Part print with two shaded views. Sizes in mm from the minimum x, y, z corner. Give positions to 0.01 mm unless a question says otherwise; leave off trailing zeros. Loops run counter-clockwise (first coordinate to the right, second up) from the corner with the lowest first, then second, coordinate; pieces in that order, holes last. Notation, with made-up numbers: M -38.75,-20 L -26.75,-20 A19 ccw -26.75,-12 Z; hole C 29.5,50 d6. An arc over 180 degrees is marked long. Answer as a JSON object with one key per item and string values. Group by question number.
1. Mould opens along X. For the marked faces 1, 2 and 3 say: released by +X, released by -X, zero draft, split by the parting line, or undercut.
2. Drop a flat-ended pin along its axis: pin 1 Ø1.5 at (x, y) = (3.5, 55) entering from -Z. Give the stop position or say it passes through.
3. Slice it at D-D (x = 3). List the corners of the cut face in (y, z).
4. Slice it at C-C (x = 6). List the corners of the cut face in (y, z).
5. Slice it at A-A (y = 66). List the corners of the cut face in (x, z).
6. Slice it at B-B (z = 5.2). List the corners of the cut face in (x, y), then the cut area to 3 significant figures.
7. Drill centre lines: line 1 along Y through (x, z) = (6, 2); line 2 along Y through (x, z) = (4, 1.25); line 3 along X through (y, z) = (66, 4.25). Where is each one in solid material? Low to high. Write a range as [from, to].
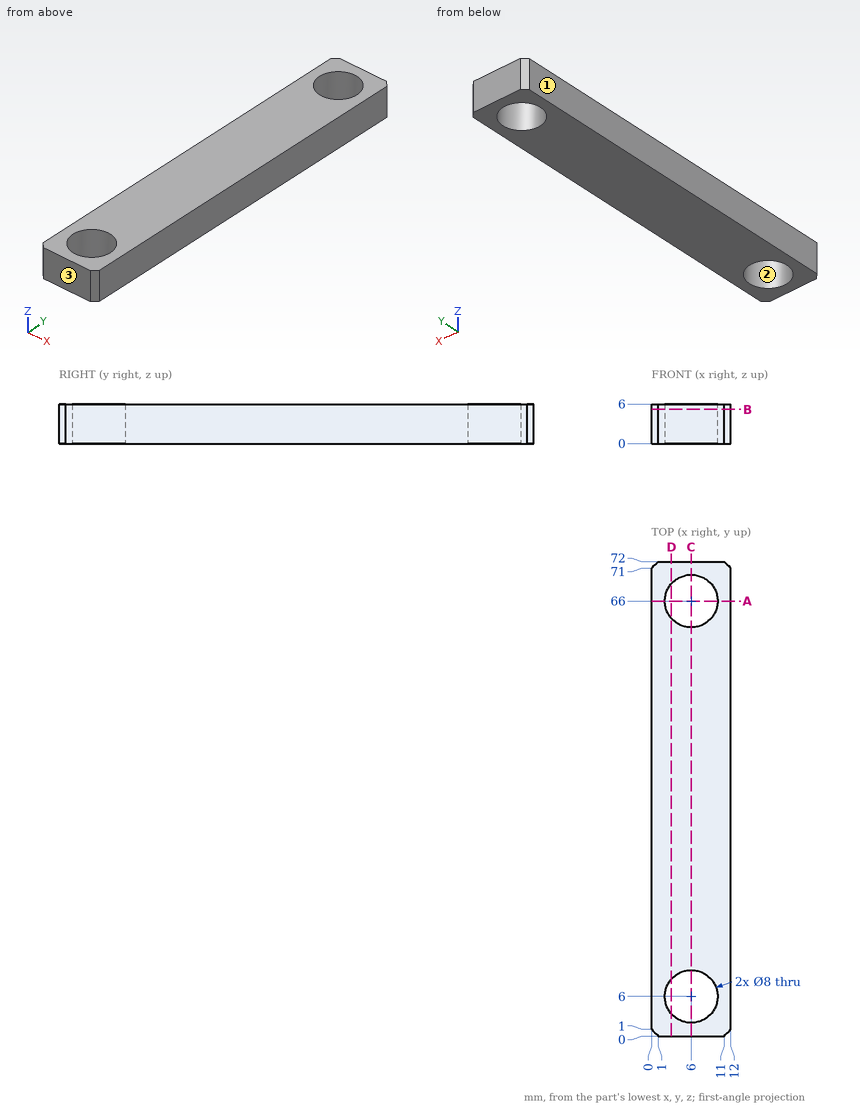
Established:
{
 "1": {"face 1": "released by -X", "face 2": "undercut", "face 3": "zero draft"},
 "2": {"pin 1": "stops at z = 0"},
 "3": {"outline": "M 0,0 L 3.35,0 L 3.35,6 L 0,6 Z; M 8.65,0 L 63.35,0 L 63.35,6 L 8.65,6 Z; M 68.65,0 L 72,0 L 72,6 L 68.65,6 Z"},
 "4": {"outline": "M 0,0 L 2,0 L 2,6 L 0,6 Z; M 10,0 L 62,0 L 62,6 L 10,6 Z; M 70,0 L 72,0 L 72,6 L 70,6 Z"},
 "5": {"outline": "M 0,0 L 2,0 L 2,6 L 0,6 Z; M 10,0 L 12,0 L 12,6 L 10,6 Z"},
 "6": {"outline": "M 0,1 L 1,0 L 11,0 L 12,1 L 12,71 L 11,72 L 1,72 L 0,71 Z; hole C 6,6 d8; hole C 6,66 d8", "area": "761 mm^2"},
 "7": {"line 1": "y = [0, 2], [10, 62], [70, 72]", "line 2": "y = [0, 2.54], [9.46, 62.54], [69.46, 72]", "line 3": "x = [0, 2], [10, 12]"}
}
